Part model, mm, in its own coordinate system. Face numbers are marked on the shaded views. Coordinates: 2 decimals unless noted, no trailing zeros. Write each loop counter-clockwise with the first axis right and the second up, starting at its lowest first coordinate (ties: lowest second). Pieces come first, ordered by that corner, then holes. Notation, with made-up numbers: (10, -21.75) - (46, -21.75) arc R25 ccw to (46, 10.25) - close; hole circle Ø6 at (64.5, 76.25). An arc over 180 degrees is marked (long way). Use a Markdown table: item, result.
Autodesk Inventor part; units mm, degrees
ref_plane "YZ Plane" through (0, 0, 0) normal (1, 0, 0) x (0, 1, 0)
ref_plane "XZ Plane" through (0, 0, 0) normal (0, 1, 0) x (-1, 0, 0)
ref_plane "XY Plane" through (0, 0, 0) normal (0, 0, 1) x (1, 0, 0)
sketch "Sketch1" plane through (0, 0, 0) normal (0, 0, 1) x (1, 0, 0)
  line L0 (8.25, 5) -> (-8.25, 5)
  line L1 (-8.25, 5) -> (-8.25, -5)
  line L2 (-8.25, -5) -> (8.25, -5)
  line L3 (8.25, -5) -> (8.25, 5)
  point P0 (0, 0)
  dimension "d19" = 10
  dimension "d36" = 16.5
  dimension "d37" = 5
extrude "Box" add sketch "Sketch1" along normal blind 6.927 and the other way blind 6.223
sketch "Sketch3" plane through (0, 0, -6.223) normal (0, 0, -1) x (-1, 0, 0)
  line L0 (-5.08, 0) -> (5.08, 0) construction
  line L1 (-4.75, 0) -> (4.75, 0) construction
  circle A0 centre (0, 0) radius 2
  dimension "d35" = 4
extrude "Slot" cut sketch "Sketch3" against normal blind 11.15
sketch "Sketch4" plane through (0, 0, -6.223) normal (0, 0, -1) x (-1, 0, 0)
  circle A0 centre (-2.96, 3.0769) radius 1.45
  line L0 (8.25, 5) -> (-8.25, 5)
  circle A1 centre (0, 0) radius 2
  line L1 (-8.25, 5) -> (-8.25, -5)
  dimension "d32" = 2.9
  dimension "d34" = 1.9231
  dimension "d39" = 5.29
  dimension "d40" = 5
extrude "MountingHole" cut sketch "Sketch4" against normal blind 15 contours A0
pattern_linear "Mounting Holes" count 2 spacing 5.92 along (-1, 0, 0) count 2 spacing 6.154 along (0, -1, 0) of "MountingHole"
sketch "Sketch6" plane through (-8.25, 5, 6.927) normal (0, 1, 0) x (1, 0, 0)
  circle A0 centre (8.25, 9.65) radius 1.105
  line L0 (0, 13.15) -> (16.5, 13.15)
  dimension "d20" = 2.21
  dimension "d46" = 3.5
extrude "CentralSMAHole" cut sketch "Sketch6" against normal blind 12
sketch "Sketch8" plane through (-8.25, 5, 6.927) normal (0, 1, 0) x (1, 0, 0)
  circle A0 centre (14.36, 9.65) radius 1.295
  line L0 (0, 13.15) -> (16.5, 13.15)
  dimension "d23" = 2.59
  dimension "d45" = 3.5
extrude "SMAMounting" cut sketch "Sketch8" against normal blind 12
pattern_linear "SMAMountingHoles" count 2 spacing 12.22 along (-1, 0, 0) of "SMAMounting"
equation "\"d34\" = 0.384615 * d40"
properties part number "NewSinkV3"
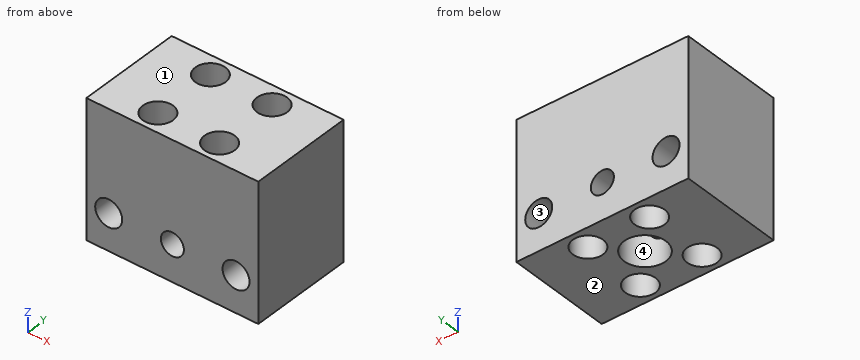
Item 1: Band-saw the part on B-B, the plane x = 6.11. Give the cut face in (y, z).
From the geometry:
| item | result |
|---|---|
| outline | (-5, -6.22) - (5, -6.22) - (5, -4.02) - (-5, -4.02) - close; (-5, -1.43) - (5, -1.43) - (5, 6.93) - (-5, 6.93) - close |
Item 2: Drop a flat-ended pin along its axis: P1, Ø1.2, axis at x = 1, y = 0.5, coming from the -Z side. Give the stop position or say it passes through.
From the geometry:
| item | result |
|---|---|
| P1 | z = 4.93 |
Item 3: Band-saw the part on A-A, the plane x = -2.96. Give the cut face in (y, z).
From the geometry:
| item | result |
|---|---|
| outline | (-5, -6.22) - (-4.53, -6.22) - (-4.53, 6.93) - (-5, 6.93) - close; (-1.63, -6.22) - (1.63, -6.22) - (1.63, 6.93) - (-1.63, 6.93) - close; (4.53, -6.22) - (5, -6.22) - (5, 6.93) - (4.53, 6.93) - close |
Item 4: Two-plate mould, pull along Z, no slides. Class the marked faces 1, 2, 3 and 4: pulls with the +Z half, pulls with the -Z half, needs draft (parallel to the pull), parting line crosses it, or undercut.
From the geometry:
| item | result |
|---|---|
| face 1 | pulls with the +Z half |
| face 2 | pulls with the -Z half |
| face 3 | undercut |
| face 4 | needs draft |
Item 5: Drill centre lines: probe 1 along Y at (x, z) = (2.96, 2.5); probe 2 along X at (y, z) = (-3.25, 4.5); probe 3 along Z at (x, y) = (-6.11, -1.75). Where is each one in solid material? Low to high.
From the geometry:
| item | result |
|---|---|
| probe 1 | -5 to -4.53, -1.63 to 1.63, 4.53 to 5 |
| probe 2 | -8.25 to -4.4, -1.52 to 1.52, 4.4 to 8.25 |
| probe 3 | -6.22 to -4.02, -1.43 to 6.93 |
Item 6: Band-saw the part on D-D, the plane y = 1. Give the cut face in (x, z) (3 decimals).
From the geometry:
| item | result |
|---|---|
| outline | (-8.25, -6.223) - (-1.732, -6.223) - (-1.732, 4.927) - (1.732, 4.927) - (1.732, -6.223) - (8.25, -6.223) - (8.25, 6.927) - (-8.25, 6.927) - close; hole circle Ø2.59 at (-6.11, -2.723); hole circle Ø2.59 at (6.11, -2.723) |
Item 7: Band-saw the part on C-C, the plane z = 1.5. Give the cut face in (x, y).
From the geometry:
| item | result |
|---|---|
| outline | (-8.25, -5) - (8.25, -5) - (8.25, 5) - (-8.25, 5) - close; hole circle Ø2.9 at (-2.96, -3.08); hole circle Ø2.9 at (-2.96, 3.08); hole circle Ø4 at (0, 0); hole circle Ø2.9 at (2.96, -3.08); hole circle Ø2.9 at (2.96, 3.08) |
